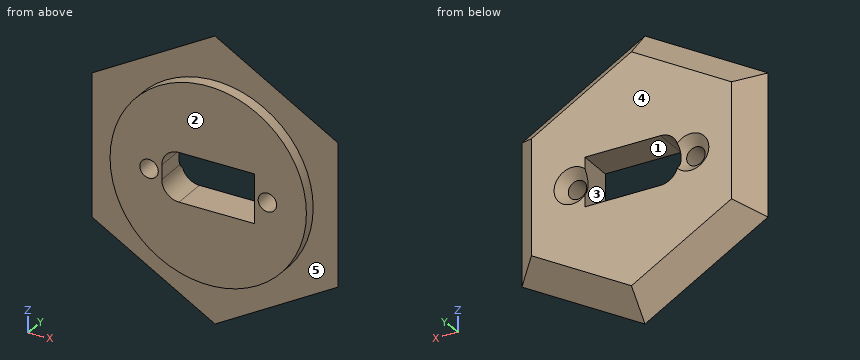
```python
from build123d import *

# Parameters (mm, degrees)
SKETCH1_R                                           = 26
BOSS_EXTRUDE1_DEPTH                                 = 4
SKETCH3_R                                           = 17
BOSS_EXTRUDE2_DEPTH                                 = 2
CUT_EXTRUDE1_DEPTH                                  = 20
SKETCH4_R                                           = 1.6
CUT_EXTRUDE2_DEPTH                                  = 10
SKETCH6_OUTSIDE_W                                   = 88.756
SKETCH6_OUTSIDE_H                                   = 88.756
CUT_EXTRUDE3_DEPTH                                  = 10
CUT_EXTRUDE3_TAPER                                  = 45
CSK_FOR_M3_COUNTERSUNK_FLAT_HEAD_SCREW2_D           = 3.2
CSK_FOR_M3_COUNTERSUNK_FLAT_HEAD_SCREW2_CSINK_D     = 6.3
CSK_FOR_M3_COUNTERSUNK_FLAT_HEAD_SCREW2_CSINK_ANGLE = 90


with BuildPart() as part:
    # Sketch1 → Boss-Extrude1 (new body)
    with BuildSketch(Plane(origin=(0, 0, 0), x_dir=(1, 0, 0), z_dir=(0, 1, 0))):
        Circle(SKETCH1_R)
    extrude(amount=BOSS_EXTRUDE1_DEPTH)

    # Sketch3 → Boss-Extrude2 (add)
    with BuildSketch(Plane.XZ):
        Circle(SKETCH3_R)
    extrude(amount=BOSS_EXTRUDE2_DEPTH)

    # Sketch2 → Cut-Extrude1 (cut)
    with BuildSketch(Plane(origin=(0, 4, 0), x_dir=(1, 0, 0), z_dir=(0, 1, 0))):
        with BuildLine():
            Line((-5.05, -4.25), (8.05, -4.25))
            Line((8.05, -4.25), (8.05, 4.25))
            Line((8.05, 4.25), (-5.05, 4.25))
            ThreePointArc((-5.05, 4.25), (-7.171320344, 3.371320344), (-8.05, 1.25))
            Line((-8.05, 1.25), (-8.05, -1.25))
            ThreePointArc((-8.05, -1.25), (-7.171320344, -3.371320344), (-5.05, -4.25))
        make_face()
    extrude(amount=-CUT_EXTRUDE1_DEPTH, mode=Mode.SUBTRACT)

    # Sketch4 → Cut-Extrude2 (cut)
    with BuildSketch(Plane(origin=(0, 4, 0), x_dir=(1, 0, 0), z_dir=(0, 1, 0))):
        with Locations((-10.25, 0)):
            Circle(SKETCH4_R)
        with Locations((10.25, 0)):
            Circle(SKETCH4_R)
    extrude(amount=-CUT_EXTRUDE2_DEPTH, mode=Mode.SUBTRACT)

    # Sketch6 outside → Cut-Extrude3 (cut)
    with BuildSketch(Plane(origin=(0, 4, 0), x_dir=(1, 0, 0), z_dir=(0, 1, 0))):
        Rectangle(SKETCH6_OUTSIDE_W, SKETCH6_OUTSIDE_H)
        Polygon((0, 20), (-17.320508076, 10), (-17.320508076, -10), (0, -20), (17.320508076, -10), (17.320508076, 10), align=None, mode=Mode.SUBTRACT)
    extrude(amount=-CUT_EXTRUDE3_DEPTH, taper=CUT_EXTRUDE3_TAPER, mode=Mode.SUBTRACT)

    # CSK for M3 Countersunk Flat Head Screw2 (through all)
    with Locations(Plane(origin=(0, 4, 0), x_dir=(1, 0, 0), z_dir=(0, 1, 0))):
        with Locations((-10.25, 0), (10.25, 0)):
            CounterSinkHole(CSK_FOR_M3_COUNTERSUNK_FLAT_HEAD_SCREW2_D / 2, CSK_FOR_M3_COUNTERSUNK_FLAT_HEAD_SCREW2_CSINK_D / 2, counter_sink_angle=CSK_FOR_M3_COUNTERSUNK_FLAT_HEAD_SCREW2_CSINK_ANGLE)


solid = part.part
```
The listing builds one solid part. Answer for the finished solid, in the listing's coordinates (mm). Face numbers are marked on the shaded views. A direction names the side the tool comes from. Round coordinates to 2 decimals unless told otherwise and drop trailing zeros.
Q1. Which of the six approach directions +Z, -Z, +X, -X, +Y, -Y give full straight-line access (tool end or side, diameter ignored) to the marked faces 3, 4 and 5?
Q2. For a pull along Z with two mould halves and no side action, classify the marked faces 1 and 2 as released by +Z, released by -Z, zero draft, split by the parting line, or undercut.
Q3. Section A-A, the plane z = 0 is taken. Count the separate pieces of the cut face and the enclosed holes in it, then the cut area to 3 significant figures.
Q4. Given pin 1 Ø4 at (x, z) = (-10.25, 0) entering from +Y; pin 2 Ø1.5 at (x, z) = (8.5, 18.5) entering from +Y; pin 3 Ø2 at (y, z) = (2, 0.5) entering from +X, each flat-ended and moving along its own axis, determine where each tip first touches the part or whether it passes through.
Q5. Find the intervals of material crossed by line 1 (X direction, y = 1.2, z = 0); line 2 (X direction, y = 0.35, z = 0); line 3 (Z direction, x = -10, y = 0.5), in increasing order.
Completed:
1. face 3: +Y, -Y
1. face 4: +Z, -Z, +X, -X, +Y
1. face 5: -Y
2. face 1: undercut
2. face 2: zero draft
3. separate pieces: 4
3. enclosed holes: 0
3. area: 83.7 mm2
4. pin 1: stops at y = 2.85
4. pin 2: stops at y = 1.8
4. pin 3: stops at x = 20.32
5. line 1: x = -20.12 to -11.85, -8.65 to -8.05, 8.05 to 8.65, 11.85 to 20.12
5. line 2: x = -20.97 to -11.85, -8.65 to -8.05, 8.05 to 8.65, 11.85 to 20.97
5. line 3: z = -18.27 to -1.58, 1.58 to 18.27
